from build123d import *

# Parameters (mm, degrees)
CUT_EXTRUDE1_DEPTH = 21
CUT_EXTRUDE2_DEPTH = 2
SKETCH3_R          = 1.475
CUT_EXTRUDE3_DEPTH = 8.9
CUT_EXTRUDE4_START = -2.8
SKETCH3_4_R        = 3
SKETCH3_4_R_2      = 1.475
CUT_EXTRUDE4_DEPTH = 6.1
CUT_EXTRUDE5_DEPTH = 2


with BuildPart() as part:
    # Sketch1 → Revolve1 (revolve)
    with BuildSketch(Plane(origin=(0, 0, 0), x_dir=(1, 0, 0), z_dir=(0, 1, 0))):
        Polygon((0, 0), (0, 11), (-7.2, 11), (-7.2, 9.2), (-59, 9.2), (-59, 0), align=None)
    revolve(axis=Axis((0, 0, 0), (-1, 0, 0)))

    # Sketch2 → Cut-Extrude1 (cut)
    with BuildSketch(Plane(origin=(0, 0, 0), x_dir=(0, 0, -1), z_dir=(1, 0, 0))):
        with BuildLine():
            Line((2.527844932, 3.1), (-2.527844932, 3.1))
            ThreePointArc((-2.527844932, 3.1), (-1.715899221, -3.613265817), (4, 0))
            ThreePointArc((4, 0), (3.613265817, 1.715899221), (2.527844932, 3.1))
        make_face()
    extrude(amount=-CUT_EXTRUDE1_DEPTH, mode=Mode.SUBTRACT)

    # Sketch2_4 → Cut-Extrude2 (cut)
    with BuildSketch(Plane(origin=(0, 0, 0), x_dir=(0, 0, -1), z_dir=(1, 0, 0))):
        with BuildLine():
            ThreePointArc((2.527844932, 3.1), (0, 4), (-2.527844932, 3.1))
            Line((-2.527844932, 3.1), (2.527844932, 3.1))
        make_face()
        with BuildLine():
            Line((2.527844932, 3.1), (-2.527844932, 3.1))
            ThreePointArc((-2.527844932, 3.1), (-1.715899221, -3.613265817), (4, 0))
            ThreePointArc((4, 0), (3.613265817, 1.715899221), (2.527844932, 3.1))
        make_face()
    extrude(amount=-CUT_EXTRUDE2_DEPTH, mode=Mode.SUBTRACT)

    # Sketch3 → Cut-Extrude3 (cut, through all)
    with BuildSketch(Plane.XZ.offset(-3.1)):
        with Locations((-14, 0)):
            Circle(SKETCH3_R)
    extrude(amount=-CUT_EXTRUDE3_DEPTH, mode=Mode.SUBTRACT)

    # Sketch3_4 → Cut-Extrude4 (cut, through all)
    with BuildSketch(Plane.XZ.offset(-3.1).offset(CUT_EXTRUDE4_START)):
        with Locations((-14, 0)):
            Circle(SKETCH3_4_R)
        with Locations((-14, 0)):
            Circle(SKETCH3_4_R_2, mode=Mode.SUBTRACT)
    extrude(amount=-CUT_EXTRUDE4_DEPTH, mode=Mode.SUBTRACT)

    # Sketch2_6 → Cut-Extrude5 (cut)
    with BuildSketch(Plane(origin=(0, 0, 0), x_dir=(0, 0, -1), z_dir=(1, 0, 0))):
        with BuildLine():
            Line((0.5, 9.488630488), (0.5, 10.988630488))
            ThreePointArc((0.5, 10.988630488), (0, 11), (-0.5, 10.988630488))
            Line((-0.5, 10.988630488), (-0.5, 9.488630488))
            Line((-0.5, 9.488630488), (0.5, 9.488630488))
        make_face()
        with BuildLine():
            ThreePointArc((-0.5, -10.988630488), (0, -11), (0.5, -10.988630488))
            Line((0.5, -10.988630488), (0.5, -9.488630488))
            Line((0.5, -9.488630488), (-0.5, -9.488630488))
            Line((-0.5, -9.488630488), (-0.5, -10.988630488))
        make_face()
    extrude(amount=-CUT_EXTRUDE5_DEPTH, mode=Mode.SUBTRACT)


solid = part.part
Read the model definition and answer for the solid it produces. Units are mm, in the model's axes. A direction names the side the tool comes from. Coordinates: 2 decimals unless noted, no trailing zeros. Loops run counter-clockwise (first coordinate to the right, second up) from the corner with the lowest first, then second, coordinate; pieces in that order, holes last. Notation, with made-up numbers: (-25, 50) -> (-14, 50) arc R20 cw to (-14, 59) -> close; hole circle Ø3 at (38, 28). An arc over 180 degrees is marked (long way). Write item = value, one per line. Start each with the question number.
1) The part is cut by section D-D, the plane x = -29. Determine the outline of the cut face in (y, z), plus the area to 3 significant figures.
2) Given P1, Ø1.5, axis at x = -17.5, z = 8.5, coming from the +Y side; P2, Ø1.5, axis at x = -50, y = 4.5, coming from the -Z side; P3, Ø0.5, axis at x = -1, y = 10, coming from the -Z side, each flat-ended and moving along its own axis, determine where each tip first touches the part or whether it passes through.
3) The part is cut by section B-B, the plane y = -6.5. Determine the outline of the cut face in (x, z).
4) Find the intervals of material crossed by L1, parallel to Y at x = -8, z = 0; L2, parallel to Z at x = -6.75, y = 0; L3, parallel to Y at x = -6.75, z = 0, in increasing order. Write a range as from..to.
5) The part is cut by section C-C, the plane x = -4.5. Determine the outline of the cut face in (y, z).
6) The mould has two halves that part along Z. Classify faces 6 (the face through (-3.65, 10.74, 2.38)), 7 (the face through (-7.2, 8, -5)), 8 (the face through (-21, 0, 0)): pulls with the +Z half, pulls with the -Z half, needs draft (parallel to the pull), parting line crosses it, or undercut.
7) The part is cut by section A-A, the plane z = 8. Determine the outline of the cut face in (x, y).
8) For faces 1 (the face through (-14.65, 7.53, -2.93)), 2 (the face through (-11, 3.1, 0)), 3 (the face through (-1, -10, -0.5)), 4 (the face through (-33.463, -7.757, -4.946)), 5 (the face through (-1, 10, -0.5)), determine the directions among +Z, -Z, +X, -X, +Y, -Y from which every point of the face is accessible in a straight line to the end or side of a thin tool.
Result:
q1.outline = circle Ø18.4 at (0, 0)
q1.area = 266 mm²
q2.P1 = 4.96
q2.P2 = -8.4
q2.P3 = -5.09
q3.outline = (-59, -6.51) -> (-7.2, -6.51) -> (-7.2, -8.87) -> (0, -8.87) -> (0, 8.87) -> (-7.2, 8.87) -> (-7.2, 6.51) -> (-59, 6.51) -> close
q4.L1 = -9.2..-4, 3.1..9.2
q4.L2 = -11..-4, 4..11
q4.L3 = -11..-4, 3.1..11
q5.outline = circle Ø22 at (0, 0); hole (3.1, -2.53) -> (3.1, 2.53) arc R4 ccw (long way) to start
q6.face_6 = parting line crosses it
q6.face_7 = needs draft
q6.face_8 = undercut
q7.outline = (-59, -4.54) -> (-7.2, -4.54) -> (-7.2, -7.55) -> (0, -7.55) -> (0, 7.55) -> (-7.2, 7.55) -> (-7.2, 4.54) -> (-59, 4.54) -> close
q8.face_1 = +Y
q8.face_2 = +X
q8.face_3 = +X, -Y
q8.face_4 = -X
q8.face_5 = +X, +Y
